from build123d import *

# Parameters (mm, degrees)
SKETCH1_W               = 300
SKETCH1_H               = 80
BOSS_EXTRUDE1_DEPTH     = 50
SKETCH2_R               = 9
CUT_EXTRUDE1_DEPTH      = 41
CUT_EXTRUDE1_DEPTH_BACK = 41


with BuildPart() as part:
    # Sketch1 → Boss-Extrude1 (new body, symmetric)
    with BuildSketch(Plane.XY):
        Rectangle(SKETCH1_W, SKETCH1_H)
    extrude(amount=BOSS_EXTRUDE1_DEPTH, both=True)

    # Sketch2 → Cut-Extrude1 (cut, two sides)
    with BuildSketch(Plane(origin=(0, 0, 0), x_dir=(1, 0, 0), z_dir=(0, 1, 0))) as cut_extrude1_sk:
        with Locations((-115, 10)):
            Circle(SKETCH2_R)
        with Locations((115, 10)):
            Circle(SKETCH2_R)
    extrude(amount=CUT_EXTRUDE1_DEPTH, mode=Mode.SUBTRACT)
    extrude(cut_extrude1_sk.sketch, amount=-CUT_EXTRUDE1_DEPTH_BACK, mode=Mode.SUBTRACT)


solid = part.part
CAD build for the part. Positions are in the model's coordinates, mm. Round coordinates to 2 decimals unless told otherwise and drop trailing zeros. Order: outer loops, then holes, each group sorted by start corner. A loop starts at its lowest first (then second) coordinate and runs counter-clockwise, first axis right, second up. Notation, with made-up numbers: (55.5, -30.5) -> (102.5, -30.5) arc R27 ccw to (102.5, -12.5) -> close; hole circle Ø11 at (35.25, -25.5). An arc over 180 degrees is marked (long way). Write item = value, one per line. Start each with the question number.
(1) Cut at C-C, the plane y = 33.5. List the corners of the cut face in (x, z).
(2) Probe line 1 (X direction, y = -23, z = -10); line 2 (Z direction, x = 115, y = 10.5); line 3 (Z direction, x = -108.5, y = -28.5). List the from-to ranges inside material, lowest first. Write a range as [from, to].
(3) Cut at B-B, the plane z = -10. List the corners of the cut face in (x, y), then the cut area to 3 significant figures.
(4) Cut at A-A, the plane x = -115. List the corners of the cut face in (y, z), then the cut area to 3 significant figures.
(5) Pull direction X, two halves, no side cores. Call faces 1 (the cylindrical face through (-106.686, 0.56, -6.553)), 2 (the flat face through (-2, 1, 50)), 3 (the flat face through (-150, -1, 1)): released by +X, released by -X, zero draft, split by the parting line, or undercut.
(6) Pin check, flat tip, straight feed: P1, Ø11, axis at x = -115, z = -10, coming from the -Y side. Stop position of the tip, or through.
Model answer:
q1.outline = (-150, -50) -> (150, -50) -> (150, 50) -> (-150, 50) -> close; hole circle Ø18 at (-115, -10); hole circle Ø18 at (115, -10)
q2.line_1 = [-150, -124], [-106, 106], [124, 150]
q2.line_2 = [-50, -19], [-1, 50]
q2.line_3 = [-50, -16.22], [-3.78, 50]
q3.outline = (-150, -40) -> (-124, -40) -> (-124, 40) -> (-150, 40) -> close; (-106, -40) -> (106, -40) -> (106, 40) -> (-106, 40) -> close; (124, -40) -> (150, -40) -> (150, 40) -> (124, 40) -> close
q3.area = 21,100 mm2
q4.outline = (-40, -50) -> (40, -50) -> (40, -19) -> (-40, -19) -> close; (-40, -1) -> (40, -1) -> (40, 50) -> (-40, 50) -> close
q4.area = 6,560 mm2
q5.face_1 = undercut
q5.face_2 = zero draft
q5.face_3 = released by -X
q6.P1 = through
